```python
from build123d import *

# Parameters (mm, degrees)
ESQUISSE1_W             = 100
ESQUISSE1_H             = 100
BOSS_EXTRU_1_DEPTH      = 5
ESQUISSE2_W             = 20
ESQUISSE2_H             = 5
ESQUISSE2_W_2           = 5
ESQUISSE2_H_2           = 18
ENL_V_MAT_EXTRU_1_DEPTH = 5


with BuildPart() as part:
    # Esquisse1 → Boss.-Extru.1 (new body)
    with BuildSketch(Plane.XY):
        with Locations((-50, -50)):
            Rectangle(ESQUISSE1_W, ESQUISSE1_H)
    extrude(amount=BOSS_EXTRU_1_DEPTH)

    # Esquisse2 → Enlèv. mat.-Extru.1 (cut)
    with BuildSketch(Plane(origin=(0, 0, 0), x_dir=(-1, 0, 0), z_dir=(0, 0, -1))):
        with Locations((70, -97.5)):
            Rectangle(ESQUISSE2_W, ESQUISSE2_H)
        with Locations((30, -97.5)):
            Rectangle(ESQUISSE2_W, ESQUISSE2_H)
        with Locations((30, -2.5)):
            Rectangle(ESQUISSE2_W, ESQUISSE2_H)
        with Locations((70, -2.5)):
            Rectangle(ESQUISSE2_W, ESQUISSE2_H)
        with Locations((97.5, -68)):
            Rectangle(ESQUISSE2_W_2, ESQUISSE2_H_2)
        with Locations((97.5, -32)):
            Rectangle(ESQUISSE2_W_2, ESQUISSE2_H_2)
        with Locations((2.5, -32)):
            Rectangle(ESQUISSE2_W_2, ESQUISSE2_H_2)
        with Locations((2.5, -68)):
            Rectangle(ESQUISSE2_W_2, ESQUISSE2_H_2)
    extrude(amount=-ENL_V_MAT_EXTRU_1_DEPTH, mode=Mode.SUBTRACT)


solid = part.part
```
Source: CAD feature listing. Evaluate the final solid. Frame: model axes, mm. A direction names the side the tool comes from. Coordinates: 2 decimals unless noted, no trailing zeros. Loops run counter-clockwise (first coordinate to the right, second up) from the corner with the lowest first, then second, coordinate; pieces in that order, holes last. Notation, with made-up numbers: (38, 12.5) -> (51, 12.5) arc R29 ccw to (51, 46.5) -> close; hole circle Ø3 at (40.25, -4.5). An arc over 180 degrees is marked (long way). One line per item, written item: value. Start each with the question number.
Q1. Contact query for flat-ended pins moving along their axis: P1, Ø2.5, axis at x = -32.5, z = 2.5, coming from the +Y side; P2, Ø1.5, axis at y = -67, z = 2.5, coming from the +X side; P3, Ø2.5, axis at x = -34.5, z = 3.5, coming from the -Y side. Output: stop coordinate, or through.
Q2. Set-up query: faces 4 (the face through (-2, -23, 2)), 5 (the face through (-80, -98, 2)), 6 (the face through (-97, -41, 2)), 7 (the face through (-80, -3, 2)), 8 (the face through (0, -89, 2)). Return all of +Z, -Z, +X, -X, +Y, -Y with unobstructed straight access to the full face (end or side cutting, diameter ignored); none if empty.
Q3. Section query A-A, the plane y = -73.5. Return the cut outline in (x, z).
Q4. Line query: line 1 along Y through (x, z) = (-24, 4.6). Output: solid intervals per line, ascending.
Q5. Mould query, pull axis X, two halves, no side actions, for faces 1 (the face through (-100, -12, 2)), 2 (the face through (-30, -5, 2)), 3 (the face through (-10, 0, 2)). Classes: pulls with the +X half, pulls with the -X half, needs draft (parallel to the pull), parting line crosses it, or undercut.
Results:
1. P1: y = -5
1. P2: x = -5
1. P3: y = -95
2. face 4: +Z, -Z, +X
2. face 5: +Z, -Z, -Y
2. face 6: +Z, -Z, -X
2. face 7: +Z, -Z, +Y
2. face 8: +Z, -Z, +X, +Y, -Y
3. outline: (-95, 0) -> (-5, 0) -> (-5, 5) -> (-95, 5) -> close
4. line 1: -95 to -5
5. face 1: pulls with the -X half
5. face 2: undercut
5. face 3: needs draft
